```python
from build123d import *

# Parameters (mm, degrees)
SKETCH023_W          = 76
SKETCH023_H          = 12
PAD007_DEPTH         = 12
SKETCH065_R          = 2.2
POCKET021_DEPTH      = 0.001
POCKET021_DEPTH_BACK = 42.001
SKETCH025_R          = 1.65
POCKET022_DEPTH      = 9.290086
POCKET022_DEPTH_BACK = 9.290086
CHAMFER004_SIZE      = 0.4


with BuildPart() as part:
    # Sketch023 → Pad007 (new body)
    with BuildSketch(Plane.YZ):
        with Locations((0, 36)):
            Rectangle(SKETCH023_W, SKETCH023_H)
    extrude(amount=PAD007_DEPTH)

    # Sketch065 → Pocket021 (cut, two sides)
    with BuildSketch(Plane.XY) as pocket021_sk:
        with Locations((6, 30)):
            Circle(SKETCH065_R)
        with Locations((6, -30)):
            Circle(SKETCH065_R)
        Polygon((10.866975, 6.950634), (13, 9.083659), (13, -5.999897), (12, -5.999897), align=None)
        Polygon((0, 5.999897), (-1, 5.999897), (-1, -9.083659), (1.133025, -6.950634), align=None)
    extrude(amount=-POCKET021_DEPTH, mode=Mode.SUBTRACT)
    extrude(pocket021_sk.sketch, amount=POCKET021_DEPTH_BACK, mode=Mode.SUBTRACT)

    # Sketch025 (on DatumPlane) → Pocket022 (cut, two sides)
    with BuildSketch(Plane(origin=(6, 0, 0), x_dir=(-0.087156, 0.996195, 0), z_dir=(0.996195, 0.087156, 0))) as pocket022_sk:
        with Locations((0, 33)):
            Circle(SKETCH025_R)
    extrude(amount=-POCKET022_DEPTH, mode=Mode.SUBTRACT)
    extrude(pocket022_sk.sketch, amount=POCKET022_DEPTH_BACK, mode=Mode.SUBTRACT)

    # Chamfer004
    chamfer004_edges = [part.edges().sort_by_distance(p)[0] for p in [
        (0, -23.041829, 42),
        (0.566512, -7.517146, 42),
        (0.566512, -0.475369, 42),
        (0, 21.999948, 42),
        (6, 38, 42),
        (12, 23.041829, 42),
        (11.433488, 7.517146, 42),
        (11.433488, 0.475369, 42),
        (12, -21.999948, 42),
        (6, -38, 42),
        (3.8, -30, 42),
        (3.8, 30, 42),
        (0, -23.041829, 30),
        (0.566512, -7.517146, 30),
        (0.566512, -0.475369, 30),
        (0, 21.999948, 30),
        (6, 38, 30),
        (12, 23.041829, 30),
        (11.433488, 7.517146, 30),
        (11.433488, 0.475369, 30),
        (12, -21.999948, 30),
        (6, -38, 30),
        (3.8, -30, 30),
        (3.8, 30, 30),
    ]]
    chamfer(chamfer004_edges, length=CHAMFER004_SIZE)


with BuildPart() as part_1:
    # Body008 placement: moved
    add(part.part.moved(Location((122.7, 0, 835))))


solid = part_1.part
```
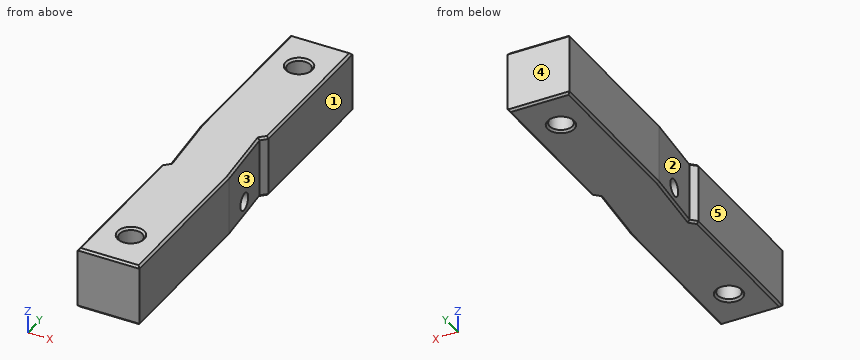
Input: part model. Units: mm. Frame: model coordinates. Face numbers are marked on the shaded views. A direction names the side the tool comes from. Give positions to 0.01 mm unless a question says otherwise; leave off trailing zeros. Write each loop counter-clockwise with the first axis right and the second up, starting at its lowest first coordinate (ties: lowest second). Pieces come first, ordered by that corner, then holes. Notation, with made-up numbers: (2.5, 72) - (26.5, 72) arc R8 ccw to (26.5, 86) - close; hole circle Ø1 at (-10, 46). An arc over 180 degrees is marked (long way). Write item = value, one per line. Start each with the question number.
1) Pin query (flat end, axial travel): pin 1 (4 mm diameter, centred on x = 128.7, y = -30, fed in from +Z). Return the tip coordinate at first contact, or that it passes through.
2) Cut plane C-C (x = 128.7). Give the number of separate pieces and of enclosed holes in the cut face, and give its area (3 significant figures).
3) Draft query along Y for the marked faces 3, 4 and 5. Return one class per face: pulls with the +Y half, pulls with the -Y half, needs draft (parallel to the pull), parting line crosses it, or undercut.
4) Material intervals for L1, parallel to Y at x = 128.7, z = 873.25; L2, parallel to Y at x = 127.75, z = 868.75; L3, parallel to Y at x = 127, z = 872.75, sorted ascending. Write a range as [from, to].
5) Cut plane B-B (y = -30). Return loops of the section in (x, z).
6) Reachability of the marked faces 1 and 2 from +Z, -Z, +X, -X, +Y, -Y: full face, straight path, thin tool, end or side. Return the list, or none.
7) Cut plane A-A (z = 872). Return loops of the section in (x, y).
Answers follow:
q1.pin_1 = through
q2.separate_pieces = 3
q2.enclosed_holes = 1
q2.area = 797 mm^2
q3.face_3 = undercut
q3.face_4 = pulls with the +Y half
q3.face_5 = needs draft
q4.L1 = [-38, -32.2], [-27.8, 27.8], [32.2, 38]
q4.L2 = [-38, -31.98], [-28.02, -1.56], [1.39, 28.02], [31.98, 38]
q4.L3 = [-38, -31.4], [-28.6, 28.6], [31.4, 38]
q5.outline = (122.7, 865.4) - (123.1, 865) - (126.1, 865) - (126.5, 865.4) - (126.5, 876.6) - (126.1, 877) - (123.1, 877) - (122.7, 876.6) - close; (130.9, 865.4) - (131.3, 865) - (134.3, 865) - (134.7, 865.4) - (134.7, 876.6) - (134.3, 877) - (131.3, 877) - (130.9, 876.6) - close
q6.face_1 = +Z, -Z, +X, +Y, -Y
q6.face_2 = +Z, -Z, -X
q7.outline = (122.7, -38) - (134.7, -38) - (134.7, -6) - (133.57, 6.95) - (134.7, 8.08) - (134.7, 38) - (122.7, 38) - (122.7, 6) - (123.83, -6.95) - (122.7, -8.08) - close; hole circle Ø4.4 at (128.7, -30); hole circle Ø4.4 at (128.7, 30)
